```python
from build123d import *

# Parameters (mm, degrees)
MODEL_R         = 1.5
MODEL_R_2       = 10
MODEL_R_3       = 2
MODEL_R_4       = 2.5
MODEL_W         = 19
MODEL_H         = 13
EXTRUDE_1_DEPTH = 2


with BuildPart() as part:
    # Model → 凸台-拉伸1 (new body)
    with BuildSketch(Plane.XY):
        with BuildLine():
            Line((347, 120), (3, 120))
            ThreePointArc((3, 120), (0.878679656, 119.121320344), (0, 117))
            Line((0, 117), (0, -117))
            ThreePointArc((0, -117), (0.878679656, -119.121320344), (3, -120))
            Line((3, -120), (347, -120))
            ThreePointArc((347, -120), (349.121320344, -119.121320344), (350, -117))
            Line((350, -117), (350, 117))
            ThreePointArc((350, 117), (349.121320344, 119.121320344), (347, 120))
        make_face()
        with Locations((4, 109.5)):
            Circle(MODEL_R, mode=Mode.SUBTRACT)
        with Locations((16, 109.5)):
            Circle(MODEL_R, mode=Mode.SUBTRACT)
        with Locations((74, 109.5)):
            Circle(MODEL_R, mode=Mode.SUBTRACT)
        with Locations((86, 109.5)):
            Circle(MODEL_R, mode=Mode.SUBTRACT)
        with Locations((194, 109.5)):
            Circle(MODEL_R, mode=Mode.SUBTRACT)
        with Locations((206, 109.5)):
            Circle(MODEL_R, mode=Mode.SUBTRACT)
        with Locations((314, 109.5)):
            Circle(MODEL_R, mode=Mode.SUBTRACT)
        with Locations((326, 109.5)):
            Circle(MODEL_R, mode=Mode.SUBTRACT)
        with Locations((5, 15)):
            Circle(MODEL_R, mode=Mode.SUBTRACT)
        with Locations((22, 15)):
            Circle(MODEL_R, mode=Mode.SUBTRACT)
        with Locations((147, 17)):
            Circle(MODEL_R, mode=Mode.SUBTRACT)
        with Locations((163, 17)):
            Circle(MODEL_R, mode=Mode.SUBTRACT)
        with Locations((308, 32)):
            Circle(MODEL_R, mode=Mode.SUBTRACT)
        with Locations((340, 32)):
            Circle(MODEL_R, mode=Mode.SUBTRACT)
        with Locations((147, -23)):
            Circle(MODEL_R, mode=Mode.SUBTRACT)
        with Locations((163, -23)):
            Circle(MODEL_R, mode=Mode.SUBTRACT)
        with Locations((340, -32)):
            Circle(MODEL_R, mode=Mode.SUBTRACT)
        with Locations((308, -32)):
            Circle(MODEL_R, mode=Mode.SUBTRACT)
        with Locations((5, -15)):
            Circle(MODEL_R, mode=Mode.SUBTRACT)
        with Locations((22, -15)):
            Circle(MODEL_R, mode=Mode.SUBTRACT)
        with Locations((326, -109.5)):
            Circle(MODEL_R, mode=Mode.SUBTRACT)
        with Locations((314, -109.5)):
            Circle(MODEL_R, mode=Mode.SUBTRACT)
        with Locations((206, -109.5)):
            Circle(MODEL_R, mode=Mode.SUBTRACT)
        with Locations((194, -109.5)):
            Circle(MODEL_R, mode=Mode.SUBTRACT)
        with Locations((4, -109.5)):
            Circle(MODEL_R, mode=Mode.SUBTRACT)
        with Locations((16, -109.5)):
            Circle(MODEL_R, mode=Mode.SUBTRACT)
        with Locations((86, -109.5)):
            Circle(MODEL_R, mode=Mode.SUBTRACT)
        with Locations((74, -109.5)):
            Circle(MODEL_R, mode=Mode.SUBTRACT)
        with Locations((116, 110)):
            Circle(MODEL_R, mode=Mode.SUBTRACT)
        with Locations((180, 110)):
            Circle(MODEL_R, mode=Mode.SUBTRACT)
        with Locations((180, 78)):
            Circle(MODEL_R, mode=Mode.SUBTRACT)
        with Locations((116, 78)):
            Circle(MODEL_R, mode=Mode.SUBTRACT)
        with Locations((116, -110)):
            Circle(MODEL_R, mode=Mode.SUBTRACT)
        with Locations((116, -78)):
            Circle(MODEL_R, mode=Mode.SUBTRACT)
        with Locations((180, -110)):
            Circle(MODEL_R, mode=Mode.SUBTRACT)
        with Locations((180, -78)):
            Circle(MODEL_R, mode=Mode.SUBTRACT)
        with Locations((65, 75)):
            Circle(MODEL_R_2, mode=Mode.SUBTRACT)
        with Locations((265, 75)):
            Circle(MODEL_R_2, mode=Mode.SUBTRACT)
        with Locations((65, -75)):
            Circle(MODEL_R_2, mode=Mode.SUBTRACT)
        with Locations((265, -75)):
            Circle(MODEL_R_2, mode=Mode.SUBTRACT)
        with Locations((196.233121438, 8.98763143)):
            Circle(MODEL_R_3, mode=Mode.SUBTRACT)
        with Locations((246.233121438, 8.98763143)):
            Circle(MODEL_R_3, mode=Mode.SUBTRACT)
        with Locations((246.233121438, -61.01236857)):
            Circle(MODEL_R_3, mode=Mode.SUBTRACT)
        with Locations((196.233121438, -61.01236857)):
            Circle(MODEL_R_3, mode=Mode.SUBTRACT)
        with Locations((57.291145141, 56.742657586)):
            Circle(MODEL_R_3, mode=Mode.SUBTRACT)
        with Locations((107.291145141, 56.742657586)):
            Circle(MODEL_R_3, mode=Mode.SUBTRACT)
        with Locations((107.291145141, -13.257342414)):
            Circle(MODEL_R_3, mode=Mode.SUBTRACT)
        with Locations((57.291145141, -13.257342414)):
            Circle(MODEL_R_3, mode=Mode.SUBTRACT)
        with Locations((223.356321923, 40.866493507)):
            Circle(MODEL_R_2, mode=Mode.SUBTRACT)
        with Locations((235.856321923, 50.866493507)):
            Circle(MODEL_R_4, mode=Mode.SUBTRACT)
        with Locations((235.856321923, 30.866493507)):
            Circle(MODEL_R_4, mode=Mode.SUBTRACT)
        with Locations((210.856321923, 50.866493507)):
            Circle(MODEL_R_4, mode=Mode.SUBTRACT)
        with Locations((210.856321923, 30.866493507)):
            Circle(MODEL_R_4, mode=Mode.SUBTRACT)
        with Locations((81.50395009, -41.835014451)):
            Circle(MODEL_R_2, mode=Mode.SUBTRACT)
        with Locations((94.00395009, -31.835014451)):
            Circle(MODEL_R_4, mode=Mode.SUBTRACT)
        with Locations((94.00395009, -51.835014451)):
            Circle(MODEL_R_4, mode=Mode.SUBTRACT)
        with Locations((69.00395009, -31.835014451)):
            Circle(MODEL_R_4, mode=Mode.SUBTRACT)
        with Locations((69.00395009, -51.835014451)):
            Circle(MODEL_R_4, mode=Mode.SUBTRACT)
        with Locations((11, 15)):
            Circle(MODEL_R, mode=Mode.SUBTRACT)
        with Locations(Location((11, -15, 0), (0, 0, 180))):
            Circle(MODEL_R, mode=Mode.SUBTRACT)
        with Locations((166.089590214, 50.675703705)):
            Rectangle(MODEL_W, MODEL_H, mode=Mode.SUBTRACT)
    extrude(amount=EXTRUDE_1_DEPTH)


solid = part.part
```
Model file for the job. Use its own axes, mm. Coordinates: 2 decimals unless noted, no trailing zeros. Order: outer loops, then holes, each group sorted by start corner. A loop starts at its lowest first (then second) coordinate and runs counter-clockwise, first axis right, second up. Notation, with made-up numbers: (11, -37.75) -> (28, -37.75) arc R17 cw to (28, -15.75) -> close; hole circle Ø10 at (21.25, 63.25). An arc over 180 degrees is marked (long way). Answer as a JSON object with one key per item and string values. Group by question number.
1) Cut at B-B, the plane z = 1.05. Count the separate pieces of the cut face and the enclosed holes in it, then the cut area to 3 significant figures.
2) Pull direction X, two halves, no side cores. Call faces 1 (the face through (86.118, -50.707, 0.986)), 2 (the face through (173, 2, 0)): +X half, -X half, draft (parallel to the pull), parting line (faces both ways), or undercut.
3) Drill centre lines: L1, parallel to Y at x = 116, z = 1.5; L2, parallel to X at y = 8.5, z = 1.65; L3, parallel to X at y = -71, z = 0.3. Where is each one in solid material? Low to high.
4) Cut at A-A, the plane y = -71. Write the cut outline in (x, z).
Check values:
{
 "1": {"separate pieces": "1", "enclosed holes": "61", "area": "81,300 mm²"},
 "2": {"face 1": "undercut", "face 2": "draft"},
 "3": {"L1": "y = -120 to -111.5, -108.5 to -79.5, -76.5 to 76.5, 79.5 to 108.5, 111.5 to 120", "L2": "x = 0 to 194.29, 198.17 to 244.29, 248.17 to 350", "L3": "x = 0 to 55.83, 74.17 to 255.83, 274.17 to 350"},
 "4": {"outline": "(0, 0) -> (55.83, 0) -> (55.83, 2) -> (0, 2) -> close; (74.17, 0) -> (255.83, 0) -> (255.83, 2) -> (74.17, 2) -> close; (274.17, 0) -> (350, 0) -> (350, 2) -> (274.17, 2) -> close"}
}
